Autodesk Inventor part; units mm, degrees
sketch "Sketch1" plane through (0, 0, 0) normal (0, 0, 1) x (1, 0, 0)
  line L0 (-6, 5) -> (6, 5) construction
  line L1 (6, 5) -> (6, -5) construction
  line L2 (6, -5) -> (-6, -5) construction
  line L3 (-6, -5) -> (-6, 5) construction
  line L4 (-6, 5) -> (6, -5) construction
  line L5 (6, 5) -> (-6, -5) construction
  line L6 (-3.5, 5) -> (3.5, 5)
  line L7 (-3.5, -5) -> (3.5, -5) construction
  arc A0 (-3.5, 5) -> (-3.5, -5) centre (-0.1834, 0) ccw
  arc A1 (3.5, -5) -> (3.5, 5) centre (0.1834, 0) ccw
  line L8 (-11.5, -5) -> (-3.5, -5)
  line L9 (3.5, -5) -> (11.5, -5)
  line L10 (-11.5, -4.8) -> (-4.1077, -4.8)
  arc A2 (-3.5598, 5.2) -> (-4.1077, -4.8) centre (-0.1834, 0) ccw
  line L11 (-3.5598, 5.2) -> (3.5598, 5.2)
  arc A3 (4.1077, -4.8) -> (3.5598, 5.2) centre (0.1834, 0) ccw
  line L12 (4.1077, -4.8) -> (11.5, -4.8)
  line L13 (11.5, -4.8) -> (11.5, -5)
  line L14 (-11.5, -4.8) -> (-11.5, -5)
  point P0 (0, 0)
  point P1 (0, 0)
  point P2 (0, 5)
  point P3 (0, 5)
  point P4 (0, -5)
  point P5 (0, -5)
  dimension "d0" = 10
  dimension "d1" = 12
  dimension "d2" = 7
  dimension "d3" = 6
  dimension "d4" = 6
  dimension "d5" = 8
  dimension "d6" = 0.2
  dimension "d11" = 7
extrude "Extrusion1" add sketch "Sketch1" along normal mid plane 10
fillet "Fillet1" radius 1 4 edges at (-11.5, -4.9, -5) (-11.5, -4.9, 5) (11.5, -4.9, 5) (11.5, -4.9, -5)
sketch "Sketch2" plane through (4.1077, -4.8, 5) normal (0, 1, 0) x (1, 0, 0)
  point P0 (-4.1077, 5)
fillet "Fillet3" radius 0.5 4 edges at (4.1077, -4.8, 0) (3.5, -5, 0) (-3.5, -5, 0) (-4.1077, -4.8, 0)
sketch "Sketch3" plane through (11.5, -4.8, 4) normal (0, 1, 0) x (1, 0, 0)
  circle A0 centre (-3.5, 1.5) radius 1
  circle A1 centre (-3.5, 6.5) radius 1
  circle A2 centre (-19.5, 6.5) radius 1
  circle A3 centre (-19.5, 1.5) radius 1
  point P0 (-11.5, 4)
extrude "Extrusion2" cut sketch "Sketch3" against normal through all
properties part number "chapa_motor_001" material "Steel"
The listing builds one solid part. Answer for the finished solid, in the listing's coordinates (mm). A direction names the side the tool comes from. Give positions to 0.01 mm unless a question says otherwise; leave off trailing zeros. Order: outer loops, then holes, each group sorted by start corner. A loop starts at its lowest first (then second) coordinate and runs counter-clockwise, first axis right, second up. Notation, with made-up numbers: (-26, 13.25) -> (-15, 13.25) arc R14 ccw to (-15, 38.25) -> close; hole circle Ø9 at (-8.75, -22.75). An arc over 180 degrees is marked (long way). Answer as a JSON object with one key per item and string values. Group by question number.
Item 1: The part is cut by section B-B on z = 2. Write down the section's boundary in (x, y).
Item 2: A tool of negligible diameter and unlimited length cuts with its end or side. For faces 1 (the cylindrical face through (6.303, 0.993, -0.07)), 2 (the cylindrical face through (-6.155, 0.587, -0.07)), from which of +Z, -Z, +X, -X, +Y, -Y can it reach the whole face along a straight path? Write none if from no direction.
Item 3: The part is cut by section D-D on z = -1. Write down the section's boundary in (x, y), and give its area (3 significant figures).
Item 4: The part is cut by section A-A on x = -8. Write down the section's boundary in (y, z).
Item 5: Determine the mould class of faces 3 (the flat face through (0, 5, 0)), 4 (the flat face through (0, 5.2, 0)), 5 (the cylindrical face through (-4.865, -4.504, -0.07)) for opening direction Y: pulls with the +Y half, pulls with the -Y half, needs draft (parallel to the pull), parting line crosses it, or undercut.
Item 6: Consider L1, parallel to Z at x = 8, y = -4.9; L2, parallel to X at y = -4.9, z = 2.5; L3, parallel to X at y = -4.85, z = 2.5. Determine where each line is inside the solid, lowest interval first. Write a range as from..to.
Item 7: Flat-ended cylindrical pins translate along their axes: pin 1 (4 mm diameter, centred on x = 0, z = 1.5, fed in from -Y); pin 2 (1.8 mm diameter, centred on x = -8, z = 2.5, fed in from -Y); pin 3 (5 mm diameter, centred on x = 9, z = -1.5, fed in from +Y); pin 4 (5.5 mm diameter, centred on x = -1, z = 2, fed in from -Y). Find the tip coordinate at first contact, or state that the pin passes through.
Item 8: The part is cut by section C-C on y = 0.5. Write down the section's boundary in (x, z).
Result set:
{
 "1": {"outline": "(-11.5, -5) -> (-8.87, -5) -> (-8.87, -4.8) -> (-11.5, -4.8) -> close; (-7.13, -5) -> (-4.87, -5) arc R0.5 ccw to (-4.51, -4.15) arc R6 cw to (-3.5, 5) -> (3.5, 5) arc R6 cw to (4.51, -4.15) arc R0.5 ccw to (4.87, -5) -> (7.13, -5) -> (7.13, -4.8) -> (5.32, -4.8) arc R0.5 cw to (4.94, -3.98) arc R6.2 ccw to (3.56, 5.2) -> (-3.56, 5.2) arc R6.2 ccw to (-4.94, -3.98) arc R0.5 cw to (-5.32, -4.8) -> (-7.13, -4.8) -> close; (8.87, -5) -> (11.5, -5) -> (11.5, -4.8) -> (8.87, -4.8) -> close"},
 "2": {"face 1": "+Z, -Z, +X", "face 2": "+Z, -Z"},
 "3": {"outline": "(-11.5, -5) -> (-4.87, -5) arc R0.5 ccw to (-4.51, -4.15) arc R6 cw to (-3.5, 5) -> (3.5, 5) arc R6 cw to (4.51, -4.15) arc R0.5 ccw to (4.87, -5) -> (11.5, -5) -> (11.5, -4.8) -> (5.32, -4.8) arc R0.5 cw to (4.94, -3.98) arc R6.2 ccw to (3.56, 5.2) -> (-3.56, 5.2) arc R6.2 ccw to (-4.94, -3.98) arc R0.5 cw to (-5.32, -4.8) -> (-11.5, -4.8) -> close", "area": "9.06 mm²"},
 "4": {"outline": "(-5, -5) -> (-4.8, -5) -> (-4.8, -3.5) -> (-5, -3.5) -> close; (-5, -1.5) -> (-4.8, -1.5) -> (-4.8, 1.5) -> (-5, 1.5) -> close; (-5, 3.5) -> (-4.8, 3.5) -> (-4.8, 5) -> (-5, 5) -> close"},
 "5": {"face 3": "pulls with the -Y half", "face 4": "pulls with the +Y half", "face 5": "undercut"},
 "6": {"L1": "-5..-3.5, -1.5..1.5, 3.5..5", "L2": "-11.5..-9, -7..-4.57, 4.57..7, 9..11.5", "L3": "-11.5..-9, -7..-4.52, 4.52..7, 9..11.5"},
 "7": {"pin 1": "y = 5", "pin 2": "through", "pin 3": "y = -4.8", "pin 4": "y = 4.82"},
 "8": {"outline": "(-6.36, -5) -> (-6.16, -5) -> (-6.16, 5) -> (-6.36, 5) -> close; (6.16, -5) -> (6.36, -5) -> (6.36, 5) -> (6.16, 5) -> close"}
}
